Part model, mm, in its own coordinate system. A direction names the side the tool comes from. Give positions to 0.01 mm unless a question says otherwise; leave off trailing zeros. Order: outer loops, then holes, each group sorted by start corner. A loop starts at its lowest first (then second) coordinate and runs counter-clockwise, first axis right, second up.
1. Slice it at C-C on z = -340. List the corners of the cut face in (x, y).
2. Slice it at D-D on y = -325. List the corners of the cut face in (x, z).
3. Mould opens along Y. For faces 1 (the flat face through (-18, -138.537, -372)), 2 (the flat face through (33.02, -206, -349)), 3 (the flat face through (-10.16, -162, -372)) say: +Y half, -Y half, draft (parallel to the pull), parting line (faces both ways), or undercut.
4. Probe line 1 (X direction, y = -271.5, z = -285.5); line 2 (Y direction, x = 35.5, z = -461.5); line 3 (X direction, y = -117, z = -51.5). List the from-to ranges inside material, lowest first.
5. Drop flat-ended pins along their axis: pin 1 Ø12 at (y, z) = (-206.5, -344) entering from +X; pin 2 Ø4 at (y, z) = (-46, -122) entering from -X; pin 3 Ø7.5 at (x, y) = (-18.5, -194) entering from +Z. Give the stop position or say it passes through.
6. Slice it at B-B on y = -266.5. List the corners of the cut face in (x, z).
7. Which spindle directions (+Z, -Z, +X, -X, +Y, -Y) get a long thin tool onto all of the face, cutting with end or side? Do faces 4 (the flat face through (-25.4, -210, -372)), 5 (the flat face through (-18, -212, -508)), 6 (the flat face through (-18, -283.012, -369)), 7 (the flat face through (19, -205, 15.264)), 8 (the flat face through (-18, -210, -232.92)). Say none if no direction does.
8. Slice it at A-A on z = -492. List the corners of the cut face in (x, y), and give its area (3 significant figures).
Autodesk Inventor part; units mm, degrees
ref_plane "YZ Plane" through (0, 0, 0) normal (1, 0, 0) x (0, 1, 0)
ref_plane "XZ Plane" through (0, 0, 0) normal (0, 1, 0) x (-1, 0, 0)
ref_plane "XY Plane" through (0, 0, 0) normal (0, 0, 1) x (1, 0, 0)
sketch "Sketch1" plane through (0, 0, 0) normal (1, 0, 0) x (0, 1, 0)
  line L0 (7.7943, 15.2638) -> (-424.0057, 15.2638)
  line L1 (-424.0057, 15.2638) -> (-424.0057, -721.3362)
  line L2 (-424.0057, -721.3362) -> (7.7943, -721.3362)
  line L3 (7.7943, -721.3362) -> (7.7943, 15.2638)
  point P0 (0, 0)
  dimension "d0" = 431.8
  dimension "d1" = 736.6
extrude "Extrusion1" add sketch "Sketch1" along normal blind 38.1
sketch "Sketch2" plane through (38.1, 0, 0) normal (1, 0, 0) x (0, 0, -1)
  line L0 (0, -9.1095) -> (708.66, -9.1095)
  line L1 (708.66, -9.1095) -> (708.66, -407.8895)
  line L2 (708.66, -407.8895) -> (0, -407.8895)
  line L3 (0, -407.8895) -> (0, -9.1095)
  point P0 (0, 0)
  dimension "d4" = 708.66
  dimension "d5" = 398.78
extrude "Extrusion2" cut sketch "Sketch2" against normal blind 5.08
sketch "Sketch3" plane through (0, 0, 0) normal (-1, 0, 0) x (0, 0, 1)
  line L0 (-470.803, -170.5411) -> (-267.603, -170.5411)
  line L1 (-267.603, -170.5411) -> (-267.603, -246.7411)
  line L2 (-267.603, -246.7411) -> (-470.803, -246.7411)
  line L3 (-470.803, -246.7411) -> (-470.803, -170.5411)
  point P0 (0, 0)
extrude "Extrusion3" add sketch "Sketch3" along normal blind 10.16
sketch "Sketch4" plane through (-10.16, 0, 0) normal (-1, 0, 0) x (0, 0, 1)
  line L0 (-508, -138.5372) -> (-232.9195, -138.5372)
  line L1 (-232.9195, -138.5372) -> (-232.9195, -283.012)
  line L2 (-232.9195, -283.012) -> (-508, -283.012)
  line L3 (-508, -283.012) -> (-508, -138.5372)
  point P0 (0, 0)
extrude "Extrusion4" add sketch "Sketch4" along normal blind 15.24
properties part number "tv1"
Data:
1. outline: (-25.4, -283.01) - (-10.16, -283.01) - (-10.16, -246.74) - (0, -246.74) - (0, -424.01) - (38.1, -424.01) - (38.1, -407.89) - (33.02, -407.89) - (33.02, -9.11) - (38.1, -9.11) - (38.1, 7.79) - (0, 7.79) - (0, -170.54) - (-10.16, -170.54) - (-10.16, -138.54) - (-25.4, -138.54) - close
2. outline: (0, -721.34) - (38.1, -721.34) - (38.1, -708.66) - (33.02, -708.66) - (33.02, 0) - (38.1, 0) - (38.1, 15.26) - (0, 15.26) - close
3. face 1: +Y half
3. face 2: undercut
3. face 3: draft
4. line 1: x = -25.4 to -10.16, 0 to 33.02
4. line 2: y = -424.01 to -407.89, -9.11 to 7.79
4. line 3: x = 0 to 33.02
5. pin 1: stops at x = 33.02
5. pin 2: stops at x = 0
5. pin 3: stops at z = -232.92
6. outline: (-25.4, -508) - (-10.16, -508) - (-10.16, -232.92) - (-25.4, -232.92) - close; (0, -721.34) - (38.1, -721.34) - (38.1, -708.66) - (33.02, -708.66) - (33.02, 0) - (38.1, 0) - (38.1, 15.26) - (0, 15.26) - close
7. face 4: +Z, -Z, -X, +Y, -Y
7. face 5: -Z, -X, +Y, -Y
7. face 6: +Z, -Z, -X, -Y
7. face 7: +Z, +X, -X, +Y, -Y
7. face 8: +Z, -X, +Y, -Y
8. outline: (-25.4, -283.01) - (-10.16, -283.01) - (-10.16, -138.54) - (-25.4, -138.54) - close; (0, -424.01) - (38.1, -424.01) - (38.1, -407.89) - (33.02, -407.89) - (33.02, -9.11) - (38.1, -9.11) - (38.1, 7.79) - (0, 7.79) - close
8. area: 16,600 mm2
